Geometry: final body of the model. Coordinates: model frame, mm. A direction names the side the tool comes from. Give positions to 0.01 mm unless a question says otherwise; leave off trailing zeros. Write each loop counter-clockwise with the first axis right and the second up, starting at its lowest first coordinate (ties: lowest second). Pieces come first, ordered by that corner, then holes.
Q1. Cut plane C-C on x = 0. Return the cut outline in (y, z).
Q2. Draft query along X for faces 4 (the face through (-0.3, 25.4, 40.5)), 5 (the face through (55.241, 13, 0)), 6 (the face through (39.992, 13, -2)). Return one class per face: pulls with the +X half, pulls with the -X half, needs draft (parallel to the pull), parting line crosses it, or undercut.
Q3. Pin query (flat end, axial travel): pin 1 (11.5 mm diameter, centred on x = 52.5, y = 12, fed in from +Z) (3 decimals); pin 2 (10 mm diameter, centred on y = 5.5, z = 21.5, fed in from -X); pin 3 (12 mm diameter, centred on x = 30.5, y = 3.5, fed in from -Z); pin 4 (3 mm diameter, centred on x = -42, z = 8.5, fed in from -Y). Return the tip coordinate at first contact, or that it passes through.
Q4. Cut plane D-D on z = 14. Return the cut outline in (x, y), plus the area to 3 significant figures.
Q5. Cut plane B-B on z = 27.5. Return the cut outline in (x, y), plus the area to 3 significant figures.
Q6. Cut plane A-A on y = 12.25. Return the cut outline in (x, z) (3 decimals).
Q7. Reachability of faces 1 (the face through (-39.992, 13, -2)), 2 (the face through (50, 13, 3.175)), 3 (the face through (-50, 13, 3.175)) from +Z, -Z, +X, -X, +Y, -Y: full face, straight path, thin tool, end or side. Return the list, or none.
Q8. Line query: L1, parallel to X at y = 20, z = 12; L2, parallel to X at y = 11.25, z = 17; L3, parallel to Z at x = 1, y = 19.25. Output: solid intervals per line, ascending.
```python
from build123d import *

# Parameters (mm, degrees)
SKETCH2_R           = 45.0723
SKETCH2_R_2         = 39.9923
BOSS_EXTRUDE1_DEPTH = 25.4
SKETCH3_W           = 90.1446
SKETCH3_H           = 25.4
CUT_EXTRUDE1_DEPTH  = 46.0723
BOSS_EXTRUDE2_DEPTH = 3.175


with BuildPart() as part:
    # Sketch2 → Boss-Extrude1 (new body)
    with BuildSketch(Plane(origin=(0, 0, 0), x_dir=(1, 0, 0), z_dir=(0, 1, 0))):
        Circle(SKETCH2_R)
        Circle(SKETCH2_R_2, mode=Mode.SUBTRACT)
    extrude(amount=BOSS_EXTRUDE1_DEPTH)

    # Sketch3 → Cut-Extrude1 (cut, through all)
    with BuildSketch(Plane.XY):
        with Locations((0, 12.7)):
            Rectangle(SKETCH3_W, SKETCH3_H)
    extrude(amount=-CUT_EXTRUDE1_DEPTH, mode=Mode.SUBTRACT)

    # Sketch5 → Boss-Extrude2 (add, symmetric)
    with BuildSketch(Plane(origin=(0, 0, 0), x_dir=(-1, 0, 0), z_dir=(0, 0, -1))):
        Polygon((-45.081415665, 25.4), (-39.9923, 25.4), (-39.9923, 0), (-45.167196058, 0), (-55.241415665, 0), (-55.241415665, 25.4), align=None)
        Polygon((45.081415665, 25.4), (55.241415665, 25.4), (55.241415665, 0), (45.167196058, 0), (39.9923, 0), (39.9923, 25.4), align=None)
    extrude(amount=BOSS_EXTRUDE2_DEPTH, both=True)


solid = part.part
```
Data:
1. outline: (0, 39.99) - (25.4, 39.99) - (25.4, 45.07) - (0, 45.07) - close
2. face 4: needs draft
2. face 5: pulls with the +X half
2. face 6: undercut
3. pin 1: stops at z = 3.175
3. pin 2: stops at x = -41.94
3. pin 3: stops at z = 16.34
3. pin 4: stops at y = 0
4. outline: (-42.84, 0) - (-37.46, 0) - (-37.46, 25.4) - (-42.84, 25.4) - close; (37.46, 0) - (42.84, 0) - (42.84, 25.4) - (37.46, 25.4) - close
4. area: 273 mm2
5. outline: (-35.71, 0) - (-29.04, 0) - (-29.04, 25.4) - (-35.71, 25.4) - close; (29.04, 0) - (35.71, 0) - (35.71, 25.4) - (29.04, 25.4) - close
5. area: 339 mm2
6. outline: (-55.241, -3.175) - (-39.992, -3.175) - (-39.992, 0) arc R39.992 cw to (39.992, 0) - (39.992, -3.175) - (55.241, -3.175) - (55.241, 3.175) - (44.96, 3.175) arc R45.072 ccw to (-44.96, 3.175) - (-55.241, 3.175) - close
7. face 1: -Z, +Y, -Y
7. face 2: +Z, +X, +Y, -Y
7. face 3: +Z, -X, +Y, -Y
8. L1: x = -43.45 to -38.15, 38.15 to 43.45
8. L2: x = -41.74 to -36.2, 36.2 to 41.74
8. L3: z = 39.98 to 45.06
